```python
from build123d import *

# Parameters (mm, degrees)
EXTRUS_O1_REACH       = 12.571
CIRPATTERN1_COUNT     = 6
FILETE1_R             = 0.3
ESBO_O24_R            = 3.35
CORTE_EXTRUS_O1_DEPTH = 0.3


with BuildPart() as part:
    # Esboço1 → Revolução1 (revolve)
    with BuildSketch(Plane.XY, mode=Mode.PRIVATE) as revolu_o1_sk:
        Polygon((0, 0), (-3.35, 0), (-3.35, 1.3), (-3.1, 1.3), (-3.05, 4.85), (-2.645980666, 6.6), (-2.65, 10.75), (0, 10.75), align=None)
    revolve(revolu_o1_sk.sketch.rotate(Axis((0, 0, 0), (0, 1, 0)), 270), axis=Axis((0, 0, 0), (0, 1, 0)))

    # Extrusão1: up to this face of the body (flat: up to its plane)
    extrus_o1_end = Plane(part.part.faces().sort_by_distance((0, 10.75, 0))[0])
    # Esboço2 → Extrusão1 (add, up to the picked face)
    with BuildSketch(Plane.XZ.offset(-1.3), mode=Mode.PRIVATE) as extrus_o1_sk1:
        with BuildLine():
            Line((-0.837606703, -2.3), (-0.204201147, -3.34377061))
            ThreePointArc((-0.204201147, -3.34377061), (0, -3.35), (0.204201147, -3.34377061))
            Line((0.204201147, -3.34377061), (0.837606703, -2.3))
            Line((0.837606703, -2.3), (-0.837606703, -2.3))
        make_face()
    extrus_o1_tool1 = split(extrude(extrus_o1_sk1.sketch, amount=-EXTRUS_O1_REACH, mode=Mode.PRIVATE), bisect_by=extrus_o1_end, keep=Keep.BOTH, mode=Mode.PRIVATE)
    add(extrus_o1_tool1.solids().sort_by(Axis((0, 1.3, -2.7171), (0, 1, 0)))[0])

    # CirPattern1: part ×6 about axis
    cirpattern1_axis = Axis((0, 0, 0), (0, 1, 0))


with BuildPart() as part_1:
    add(part.part)
    for i in range(1, CIRPATTERN1_COUNT):
        add(part.part.rotate(cirpattern1_axis, i * 360 / CIRPATTERN1_COUNT))

    # Esboço3 → Corte-Revolução5 (revolve, cut)
    with BuildSketch(Plane.XY):
        with BuildLine():
            Line((-3.2, 9.837667271), (-2.6, 10.170252702))
            ThreePointArc((-2.6, 10.170252702), (-1.331925949, 10.603305054), (0, 10.75))
            Line((0, 10.75), (0, 11.25))
            Line((0, 11.25), (-4, 11.25))
            Line((-4, 11.25), (-4, 1.3))
            Line((-4, 1.3), (-3.274507094, 1.3))
            Line((-3.274507094, 1.3), (-3.2, 9.837667271))
        make_face()
    revolve(axis=Axis((0, 0, 0), (0, 1, 0)), mode=Mode.SUBTRACT)

    # Filete1
    filete1_edges = [part_1.edges().sort_by_distance(p)[0] for p in [
        (0, 0, 3.35),
    ]]
    fillet(filete1_edges, radius=FILETE1_R)

    # Esboço24 → Corte-extrusão1 (cut)
    with BuildSketch(Plane.XZ):
        with Locations(Location((0, 0, 0), (0, 0, 270))):
            Circle(ESBO_O24_R)
    extrude(amount=-CORTE_EXTRUS_O1_DEPTH, mode=Mode.SUBTRACT)

    # Esboço22 → Revolução3 (revolve)
    with BuildSketch(Plane.XY, mode=Mode.PRIVATE) as revolu_o3_sk:
        Polygon((-0.5, 0.3), (-0.5, -0.1), (-3.079906965, -0.1), (-3.275, 0.3), align=None)
    revolve(revolu_o3_sk.sketch.rotate(Axis((0, 0, 0), (0, 1, 0)), 270), axis=Axis((0, 0, 0), (0, 1, 0)))

    # Esboço8 → Corte-Revolução6 (revolve, cut)
    with BuildSketch(Plane.XY, mode=Mode.PRIVATE) as corte_revolu_o6_sk:
        with BuildLine():
            Line((-2.808342723, -0.1), (0, -0.1))
            Line((0, -0.1), (0, 9.45))
            ThreePointArc((0, 9.45), (-1.041301106, 9.347940177), (-2.05, 9.07))
            Line((-2.05, 9.07), (-2.05, 8.47))
            ThreePointArc((-2.05, 8.47), (-1.9, 8.17), (-2.05, 7.87))
            Line((-2.05, 7.87), (-2.05, 7.37))
            Line((-2.05, 7.37), (-2.45, 5.63740965))
            Line((-2.45, 5.63740965), (-2.45, 0.45))
            ThreePointArc((-2.45, 0.45), (-2.508578644, 0.308578644), (-2.65, 0.25))
            Line((-2.65, 0.25), (-2.79, 0.25))
            Line((-2.79, 0.25), (-2.808342723, -0.1))
        make_face()
    revolve(corte_revolu_o6_sk.sketch.rotate(Axis((0, -0.1, 0), (0, 1, 0)), 270), axis=Axis((0, -0.1, 0), (0, 1, 0)), mode=Mode.SUBTRACT)


solid = part_1.part
```
Part model, mm, in its own coordinate system. A direction names the side the tool comes from. Round coordinates to 2 decimals unless told otherwise and drop trailing zeros. Order: outer loops, then holes, each group sorted by start corner. A loop starts at its lowest first (then second) coordinate and runs counter-clockwise, first axis right, second up. Notation, with made-up numbers: M 79.5,65.25 L 93.5,65.25 A34 ccw 93.5,97.25 Z; hole C -27.75,75 d7. An arc over 180 degrees is marked long. Answer in a Markdown table with one row per item. Add a question column.
Q1. Pin check, flat tips, straight feed: pin 1 (1 mm diameter, centred on y = 5.5, z = 0.5, fed in from +X); pin 2 (2.5 mm diameter, centred on x = 0, z = 0, fed in from -Y); pin 3 (2 mm diameter, centred on y = 5, z = 0.5, fed in from -X). Stop position of each tip, or through.
Q2. Cut at A-A on y = 3.5. Give the cut face in (x, z).
Q3. Mould opens along Z. For faces 1 (the face through (-2.648, 8.396, -0.01)), 2 (the face through (-1.33, 8.4, 2.29)), 3 (the face through (1.436, 5.737, -2.456)) say: +Z half, -Z half, draft (parallel to the pull), parting line (faces both ways), or undercut.
Q4. Wall check: L1, parallel to X at y = 8.9, z = 0; L2, parallel to Z at x = -0.75, y = 6.5; L3, parallel to X at y = 6.5, z = 0.25. Give the ranges that are in metal, low to high. Write a range as from..to.
Q5. 3-axis set-ups, long thin cutter, end or side, ignore diameter. For faces 4 (the face through (-3.075, 3.1, -0.017)), 5 (the face through (-0.736, 3.007, -2.337)), 6 (the face through (-2.033, 8.766, 0.267)): which of +Z, -Z, +X, -X, +Y, -Y reach the whole face in a straight line?
Established:
| question | item | result |
|---|---|---|
| 1 | pin 1 | stops at x = 2.99 |
| 1 | pin 2 | stops at y = 9.31 |
| 1 | pin 3 | stops at x = -3.06 |
| 2 | outline | M -2.94,-1.39 A3.26 ccw -2.68,-1.85 L -2.44,-1.86 A3.07 ccw -0.39,-3.04 L -0.26,-3.24 A3.26 ccw 0.26,-3.24 L 0.39,-3.04 A3.07 ccw 2.44,-1.86 L 2.68,-1.85 A3.26 ccw 2.94,-1.39 L 2.83,-1.19 A3.07 ccw 2.83,1.19 L 2.94,1.39 A3.26 ccw 2.68,1.85 L 2.44,1.86 A3.07 ccw 0.39,3.04 L 0.26,3.24 A3.26 ccw -0.26,3.24 L -0.39,3.04 A3.07 ccw -2.44,1.86 L -2.68,1.85 A3.26 ccw -2.94,1.39 L -2.83,1.19 A3.07 ccw -2.83,-1.19 Z; hole C 0,0 d4.9 |
| 3 | face 1 | undercut |
| 3 | face 2 | +Z half |
| 3 | face 3 | -Z half |
| 4 | L1 | x = -2.65..-2.05, 2.05..2.65 |
| 4 | L2 | z = -2.56..-2.12, 2.12..2.56 |
| 4 | L3 | x = -2.66..-2.24, 2.24..2.66 |
| 5 | face 4 | -X, +Y |
| 5 | face 5 | -Y |
| 5 | face 6 | none |
